Autodesk Fusion 360 part; units mm, degrees
sketch "Sketch1" plane through (0, 0, 0) normal (0, 0, 1) x (1, 0, 0)
  line L0 (0, 0) -> (0, 11)
  line L1 (0, 11) -> (11.25, 30)
  line L2 (11.25, 30) -> (11.25, 45)
  line L3 (0, 75) -> (45, 75)
  line L4 (33.75, 45) -> (33.75, 30)
  line L5 (33.75, 30) -> (45, 11)
  line L6 (45, 11) -> (45, 0)
  line L7 (45, 0) -> (0, 0)
  line L8 (11.25, 45) -> (0, 64)
  line L9 (0, 64) -> (0, 75)
  line L10 (45, 75) -> (45, 64)
  line L11 (45, 64) -> (33.75, 45)
  line L12 (-1.8, 76.8) -> (46.8, 76.8)
  line L13 (46.8, 76.8) -> (46.8, 63.5071)
  line L14 (46.8, 63.5071) -> (35.55, 44.5071)
  line L15 (35.55, 44.5071) -> (35.55, 30.4929)
  line L16 (35.55, 30.4929) -> (46.8, 11.4929)
  line L17 (46.8, 11.4929) -> (46.8, -1.8)
  line L18 (46.8, -1.8) -> (-1.8, -1.8)
  line L19 (-1.8, -1.8) -> (-1.8, 11.4929)
  line L20 (-1.8, 11.4929) -> (9.45, 30.4929)
  line L21 (9.45, 30.4929) -> (9.45, 44.5071)
  line L22 (9.45, 44.5071) -> (-1.8, 63.5071)
  line L23 (-1.8, 63.5071) -> (-1.8, 76.8)
  dimension "d1" = 75
  dimension "d2" = 45
  dimension "d3" = 45
  dimension "d4" = 11
  dimension "d5" = 11
  dimension "d7" = 30
  dimension "d8" = 30
  dimension "d9" = 30
  dimension "d10" = 30
  dimension "d13" = 11.25
  dimension "d14" = 90
  dimension "d15" = 11
  dimension "d16" = 11
  dimension "d17" = 11.25
  dimension "d18" = 11.25
  dimension "d19" = 1.8
  dimension "d20" = 1.8
  dimension "d21" = 1.8
  dimension "d22" = 1.8
  dimension "d24" = 1.8
  dimension "d25" = 1.8
  dimension "d26" = 1.8
  dimension "d27" = 1.8
  dimension "d28" = 1.8
  dimension "d29" = 1.8
  dimension "d30" = 1.8
  dimension "d31" = 1.8
extrude "Extrude1" add sketch "Sketch1" along normal blind 17
sketch "Sketch2" plane through (0, 0, 17) normal (0, 0, 1) x (-1, 0, 0)
  line L0 (-45, -75) -> (-45, -64)
  line L1 (-45, -64) -> (-33.75, -45)
  line L2 (-33.75, -45) -> (-33.75, -30)
  line L3 (-33.75, -30) -> (-45, -11)
  line L4 (-45, -11) -> (-45, 0)
  line L5 (-45, 0) -> (0, 0)
  line L6 (0, 0) -> (0, -11)
  line L7 (0, -11) -> (-11.25, -30)
  line L8 (-11.25, -30) -> (-11.25, -45)
  line L9 (-11.25, -45) -> (0, -64)
  line L10 (0, -64) -> (0, -75)
  line L11 (0, -75) -> (-45, -75)
  line L12 (1.8, -63.5071) -> (-9.45, -44.5071)
  line L13 (-9.45, -44.5071) -> (-9.45, -30.4929)
  line L14 (-9.45, -30.4929) -> (1.8, -11.4929)
  line L15 (1.8, -11.4929) -> (1.8, 1.8)
  line L16 (1.8, 1.8) -> (-46.8, 1.8)
  line L17 (-46.8, 1.8) -> (-46.8, -11.4929)
  line L18 (-46.8, -11.4929) -> (-35.55, -30.4929)
  line L19 (-35.55, -30.4929) -> (-35.55, -44.5071)
  line L20 (-35.55, -44.5071) -> (-46.8, -63.5071)
  line L21 (-46.8, -63.5071) -> (-46.8, -76.8)
  line L22 (-46.8, -76.8) -> (1.8, -76.8)
  line L23 (1.8, -76.8) -> (1.8, -63.5071)
  line L24 (1.8, -76.8) -> (1.8, -63.5071)
  line L25 (-9.45, -44.5071) -> (-9.45, -30.4929)
  line L26 (1.8, -11.4929) -> (1.8, 1.8)
  line L27 (-46.8, 1.8) -> (-46.8, -11.4929)
  line L28 (-35.55, -30.4929) -> (-35.55, -44.5071)
  line L29 (-46.8, -63.5071) -> (-46.8, -76.8)
extrude "Extrude2" add sketch "Sketch2" along normal blind 1.5 contours L0 L1 L2 L3 L4 L5 L6 L7 L8 L9 L10 L11 | L12 L13 L14 L15 L16 L17 L18 L19 L20 L21 L22 L23 L24 L25 L26 L27 L28 L29
sketch "Sketch3" plane through (0, 0, 17) normal (0, 0, -1) x (1, 0, 0)
  line L0 (0, -75) -> (45, -75)
  line L1 (45, -75) -> (45, -64)
  line L2 (45, -64) -> (33.75, -45)
  line L3 (33.75, -45) -> (33.75, -30)
  line L4 (33.75, -30) -> (45, -11)
  line L5 (45, -11) -> (45, 0)
  line L6 (45, 0) -> (0, 0)
  line L7 (0, 0) -> (0, -11)
  line L8 (0, -11) -> (11.25, -30)
  line L9 (11.25, -30) -> (11.25, -45)
  line L10 (11.25, -45) -> (0, -64)
  line L11 (0, -64) -> (0, -75)
  line L12 (8.95, -17.7) -> (16.45, -17.7)
  line L13 (16.45, -17.7) -> (16.45, -26.2)
  line L14 (16.45, -26.2) -> (8.95, -26.2)
  line L15 (8.95, -26.2) -> (8.95, -17.7)
  line L16 (9.45, -30.4929) -> (9.45, -44.5071)
  line L17 (29.55, -16.7) -> (36.55, -16.7)
  line L18 (36.55, -16.7) -> (36.55, -23.7)
  line L19 (36.55, -23.7) -> (29.55, -23.7)
  line L20 (29.55, -23.7) -> (29.55, -16.7)
  line L21 (46.8, 1.8) -> (-1.8, 1.8)
  line L22 (46.8, -11.4929) -> (46.8, 1.8)
  dimension "d37" = 8.5
  dimension "d38" = 7.5
  dimension "d43" = 25.5
  dimension "d44" = 17.25
  dimension "d45" = 7
  dimension "d46" = 7
  dimension "d49" = 0.5
  dimension "d50" = 28
extrude "Extrude3" cut sketch "Sketch3" against normal blind 7 contours L8 L14 L15 | L8 L12 L13 L14 L15 | L17 L18 L19 L20
sketch "Sketch4" plane through (0, 0, 0) normal (0, 0, -1) x (1, 0, 0)
  line L0 (45, -64) -> (45, -75)
  line L1 (45, -75) -> (0, -75)
  line L2 (0, -75) -> (0, -64)
  line L3 (0, -64) -> (11.25, -45)
  line L4 (11.25, -45) -> (11.25, -30)
  line L5 (11.25, -30) -> (0, -11)
  line L6 (0, -11) -> (0, 0)
  line L7 (0, 0) -> (45, 0)
  line L8 (45, 0) -> (45, -11)
  line L9 (45, -11) -> (33.75, -30)
  line L10 (33.75, -30) -> (33.75, -45)
  line L11 (33.75, -45) -> (45, -64)
  line L12 (9.45, -44.5071) -> (-1.8, -63.5071)
  line L13 (-1.8, -63.5071) -> (-1.8, -76.8)
  line L14 (-1.8, -76.8) -> (46.8, -76.8)
  line L15 (46.8, -76.8) -> (46.8, -63.5071)
  line L16 (46.8, -63.5071) -> (35.55, -44.5071)
  line L17 (35.55, -44.5071) -> (35.55, -30.4929)
  line L18 (35.55, -30.4929) -> (46.8, -11.4929)
  line L19 (46.8, -11.4929) -> (46.8, 1.8)
  line L20 (46.8, 1.8) -> (-1.8, 1.8)
  line L21 (-1.8, 1.8) -> (-1.8, -11.4929)
  line L22 (-1.8, -11.4929) -> (9.45, -30.4929)
  line L23 (9.45, -30.4929) -> (9.45, -44.5071)
  line L24 (9.45, -30.4929) -> (11.25, -30.4929)
  line L25 (11.25, -30.4929) -> (11.25, -44.5071)
  line L26 (11.25, -44.5071) -> (9.45, -44.5071)
  line L27 (9.45, -44.5071) -> (9.45, -30.4929)
  line L28 (35.55, -30.4929) -> (33.75, -30.4929)
  line L29 (33.75, -30.4929) -> (33.75, -44.4721)
  line L30 (33.75, -44.4721) -> (35.55, -44.4721)
  line L31 (35.55, -44.4721) -> (35.55, -30.4929)
extrude "Extrude4" add sketch "Sketch4" along normal blind 6.5 contours L10 L17 L28 L29 L30 L31 | L4 L23 L24 L25 L26 L27
Design review of the part built by this model. Coordinates are the model's own, in mm. A direction names the side the tool comes from. Give positions to 0.01 mm unless a question says otherwise; leave off trailing zeros. Order: outer loops, then holes, each group sorted by start corner. A loop starts at its lowest first (then second) coordinate and runs counter-clockwise, first axis right, second up. Notation, with made-up numbers: (-18.5, -16) - (33.5, -16) arc R18 cw to (33.5, 0) - close; hole circle Ø11 at (58, -33). An arc over 180 degrees is marked (long way). Write item = value, one per line. Start each with the question number.
Q1. Clearance check with flat-ended pins moving along their axes: pin 1 Ø3 at (y, z) = (39.5, 15.5) entering from +X; pin 2 Ø2 at (x, z) = (35, -2.5) entering from -Y; pin 3 Ø9.5 at (x, y) = (19.5, 63) entering from -Z. State where each tip first meets the part, or that it passes through.
Q2. We need section D-D on y = 40. State the section outline as (x, z) points.
Q3. To check wall thickness, follow L1, parallel to Y at x = 16, z = 11.5; L2, parallel to X at y = 36, z = 0; L3, parallel to Y at x = 5, z = 11. State the ranges of each line that lie inside material, in increasing order. Write a range as from..to.
Q4. We need section B-B on x = 40. State the section outline as (y, z) points.
Q5. Tool access review of faces 4 (the face through (45, 6, 8)), 5 (the face through (16.45, 22, 18)), 6 (the face through (3.746, 20.86, 9.12)), 7 (the face through (10, 44.507, -3)), 8 (the face through (-1.8, 70, 9)): name each direction out of +Z, -Z, +X, -X, +Y, -Y from which nothing blocks a thin tool from reaching the whole face with its end or side.
Q6. Mouldability with a two-part tool opening along X and no side actions: class faces 1 (the face through (10, 30.493, -3)), 2 (the face through (35.55, 38, 6)), 3 (the face through (29.55, 20, 18)) as released by +X, released by -X, zero draft, split by the parting line, or undercut.
Q7. We need section A-A on z = 9.25. State the section outline as (x, y) points, plus the area to 3 significant figures.
Q8. We need section C-C on x = 27. State the section outline as (y, z) points, plus the area to 3 significant figures.
Working result:
q1.pin_1 = 35.55
q1.pin_2 = 30.49
q1.pin_3 = 17
q2.outline = (9.45, -6.5) - (11.25, -6.5) - (11.25, 17) - (33.75, 17) - (33.75, -6.5) - (35.55, -6.5) - (35.55, 18.5) - (9.45, 18.5) - close
q3.L1 = -1.8..0, 75..76.8
q3.L2 = 9.45..11.25, 33.75..35.55
q3.L3 = -1.8..0, 19.44..22.98, 52.02..55.56, 75..76.8
q4.outline = (-1.8, 0) - (0, 0) - (0, 17) - (19.44, 17) - (19.44, 0) - (22.98, 0) - (22.98, 18.5) - (-1.8, 18.5) - close; (52.02, 0) - (55.56, 0) - (55.56, 17) - (75, 17) - (75, 0) - (76.8, 0) - (76.8, 18.5) - (52.02, 18.5) - close
q5.face_4 = -Z
q5.face_5 = +Z, -Z
q5.face_6 = +Z, -Z, -X
q5.face_7 = -Z, +X, -X, +Y
q5.face_8 = +Z, -Z, -X, +Y, -Y
q6.face_1 = zero draft
q6.face_2 = released by +X
q6.face_3 = undercut
q7.outline = (-1.8, -1.8) - (46.8, -1.8) - (46.8, 11.49) - (35.55, 30.49) - (35.55, 44.51) - (46.8, 63.51) - (46.8, 76.8) - (-1.8, 76.8) - (-1.8, 63.51) - (9.45, 44.51) - (9.45, 30.49) - (-1.8, 11.49) - close; hole (0, 0) - (45, 0) - (45, 11) - (33.75, 30) - (33.75, 45) - (45, 64) - (45, 75) - (0, 75) - (0, 64) - (11.25, 45) - (11.25, 30) - (0, 11) - close
q7.area = 467 mm²
q8.outline = (-1.8, 0) - (0, 0) - (0, 17) - (75, 17) - (75, 0) - (76.8, 0) - (76.8, 18.5) - (-1.8, 18.5) - close
q8.area = 179 mm²
